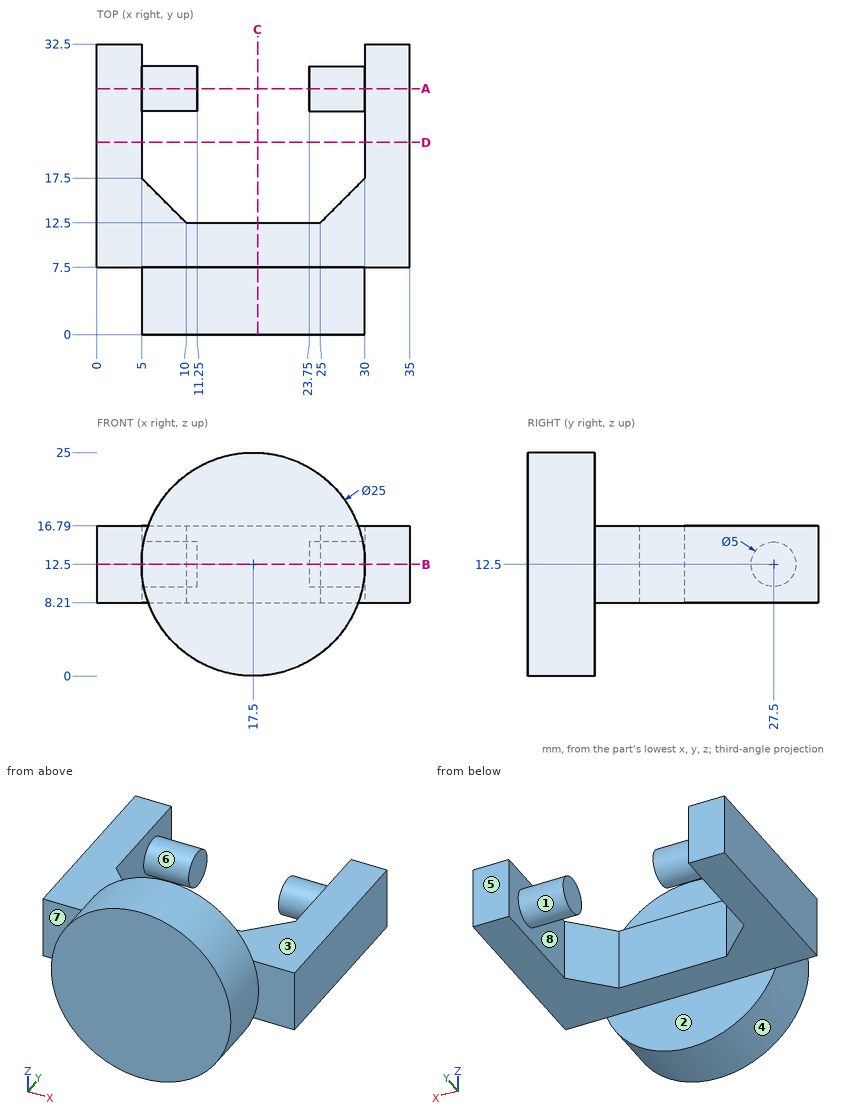
Geometry: see drawing. Coordinates: mm, zero at the bounding-box minimum. A direction names the side the tool comes from. Round coordinates to 2 decimals unless told otherwise and drop trailing zeros. Order: outer loops, then holes, each group sorted by start corner. A loop starts at its lowest first (then second) coordinate and runs counter-clockwise, first axis right, second up. Notation, with made-up numbers: (23, 2.5) -> (68, 2.5) arc R20 cw to (68, 29.5) -> close; hole circle Ø3 at (22, 53.25). An arc over 180 degrees is marked (long way). Use CSV: the item, a comma, the result in double quotes.
(1) Section B-B on z = 12.5. Return the cut outline in (x, y), and give its area (3 significant figures).
Report:
outline,"(0, 7.5) -> (5, 7.5) -> (5, 0) -> (30, 0) -> (30, 7.5) -> (35, 7.5) -> (35, 32.5) -> (30, 32.5) -> (30, 30) -> (23.75, 30) -> (23.75, 25) -> (30, 25) -> (30, 17.5) -> (25, 12.5) -> (10, 12.5) -> (5, 17.5) -> (5, 25) -> (11.25, 25) -> (11.25, 30) -> (5, 30) -> (5, 32.5) -> (0, 32.5) -> close"
area,"650 mm^2"
(2) Pull-direction query (Y, two-part tool) for the marked faces 5, 6, 7 and 8; classes: +Y half, -Y half, draft (parallel to the pull), parting line (faces both ways), or undercut.
Report:
face 5,"+Y half"
face 6,"undercut"
face 7,"-Y half"
face 8,"undercut"
(3) Section C-C on x = 18. Return the cut outline in (y, z), and give its area (3 significant figures).
Report:
outline,"(0, 0.01) -> (7.5, 0.01) -> (7.5, 8.21) -> (12.5, 8.21) -> (12.5, 16.79) -> (7.5, 16.79) -> (7.5, 24.99) -> (0, 24.99) -> close"
area,"230 mm^2"
(4) Section D-D on y = 21.5. Return the cut outline in (x, z).
Report:
outline,"(0, 8.21) -> (5, 8.21) -> (5, 16.79) -> (0, 16.79) -> close; (30, 8.21) -> (35, 8.21) -> (35, 16.79) -> (30, 16.79) -> close"
(5) Access query for the marked faces 1, 2, 3 and 4. Directions: +Z, -Z, +X, -X, +Y, -Y. A direction counts if a zero-diameter tool reaches every point of the face in a straight line with its end or side. Return the directions, or none.
Report:
face 1,"none"
face 2,"-Z, +X, -X, +Y"
face 3,"+Z, +X, -X, +Y"
face 4,"-Y"
(6) Ray query, L1, parallel to X at y = 18.5, z = 9; L2, parallel to X at y = 28.5, z = 13.5; L3, parallel to Y at x = 9.5, z = 3. Return the intervals inside material, ascending.
Report:
L1,"0 to 5, 30 to 35"
L2,"0 to 11.25, 23.75 to 35"
L3,"0 to 7.5"
(7) First-contact query: pin 1 Ø2.5 at (x, z) = (18, 13) entering from +Y; pin 2 Ø3 at (x, z) = (2.5, 14) entering from -Y; pin 3 Ø4 at (y, z) = (6, 6) entering from -X; pin 4 Ø7.5 at (x, y) = (17, 24.5) entering from -Z. Flat tips, straight axial feed; report the tip coordinate or a pass-through.
Report:
pin 1,"y = 12.5"
pin 2,"y = 7.5"
pin 3,"x = 5.84"
pin 4,"through"
(8) Section A-A on y = 27.5. Return the cut outline in (x, z).
Report:
outline,"(0, 8.21) -> (5, 8.21) -> (5, 10) -> (11.25, 10) -> (11.25, 15) -> (5, 15) -> (5, 16.79) -> (0, 16.79) -> close; (23.75, 10) -> (30, 10) -> (30, 8.21) -> (35, 8.21) -> (35, 16.79) -> (30, 16.79) -> (30, 15) -> (23.75, 15) -> close"
